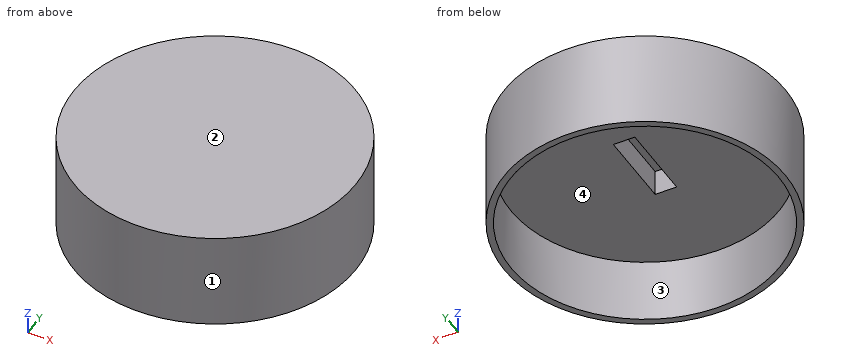
Autodesk Inventor part; units mm, degrees
ref_plane "YZ Plane" through (0, 0, 0) normal (1, 0, 0) x (0, 1, 0)
ref_plane "XZ Plane" through (0, 0, 0) normal (0, 1, 0) x (-1, 0, 0)
ref_plane "XY Plane" through (0, 0, 0) normal (0, 0, 1) x (1, 0, 0)
sketch "Esquisse1" plane through (0, 0, 0) normal (0, 0, 1) x (1, 0, 0)
  circle A0 centre (0, 0) radius 20.5
  circle A1 centre (0, 0) radius 21.5
  line L0 (0.7498, -6.187) -> (-0.7498, -6.187)
  line L1 (-0.7498, -6.187) -> (-0.7498, 6.187)
  line L2 (-0.7498, 6.187) -> (0.7498, 6.187)
  line L3 (0.7498, 6.187) -> (0.7498, -6.187)
  line L4 (0.7498, -6.187) -> (-0.7498, 6.187) construction
  line L5 (-0.7498, -6.187) -> (0.7498, 6.187) construction
  point P0 (20.5, 0)
  point P1 (21.5, 0)
  dimension "d0" = 41
  dimension "d1" = 43
  dimension "d16" = 1
extrude "Extrusion1" add sketch "Esquisse1" along normal blind 15 contours A1
sketch "Esquisse2" plane through (0, 0, 15) normal (0, 0, 1) x (1, 0, 0)
  circle A0 centre (0, 0) radius 20.5
extrude "Extrusion2" add sketch "Esquisse2" against normal blind 5
sketch "Esquisse3" plane through (0, 0, 10) normal (0, 0, -1) x (-1, 0, 0)
  line L0 (1.65, 6) -> (-1.65, 6)
  line L1 (-1.65, 6) -> (-1.65, -6)
  line L2 (-1.65, -6) -> (1.65, -6)
  line L3 (1.65, -6) -> (1.65, 6)
  line L4 (1.65, 6) -> (-1.65, -6) construction
  line L5 (-1.65, 6) -> (1.65, -6) construction
  point P0 (0, 0)
  dimension "d8" = 12
  dimension "d9" = 3.3
extrude "Extrusion3" cut sketch "Esquisse3" against normal blind 4
properties part number "Support pasApas"
Geometry check sheet. Reference: the model listing, model coordinates, mm. Face numbers are marked on the shaded views. Give positions to 0.01 mm unless a question says otherwise; leave off trailing zeros. Order: outer loops, then holes, each group sorted by start corner. A loop starts at its lowest first (then second) coordinate and runs counter-clockwise, first axis right, second up. Notation, with made-up numbers: (21, 12) - (42, 12) arc R14 cw to (42, 24) - close; hole circle Ø4 at (-33, 28). An arc over 180 degrees is marked (long way). Use one line per item in the form item = value.
1) Material ranges on probe 1 along X at (y, z) = (0.5, 8.5); probe 2 along Y at (x, z) = (0, 6.25); probe 3 along Z at (x, y) = (4.5, 15.5), recorded low to high. Write a range as from..to.
Working result:
probe_1 = -21.49..-20.49, 20.49..21.49
probe_2 = -21.5..-20.5, 20.5..21.5
probe_3 = 10..15
2) Sectioned sample at C-C (x = 0). Record the boundary of the cut face in (y, z), and give its area (3 significant figures).
Working result:
outline = (-21.5, 0) - (-20.5, 0) - (-20.5, 10) - (-6, 10) - (-6, 14) - (6, 14) - (6, 10) - (20.5, 10) - (20.5, 0) - (21.5, 0) - (21.5, 15) - (-21.5, 15) - close
area = 187 mm^2
3) Draft check along Y on the marked faces 1, 2, 3 and 4. Enter one of: released by +Y, released by -Y, zero draft, split by the parting line, or undercut.
Working result:
face_1 = split by the parting line
face_2 = zero draft
face_3 = undercut
face_4 = undercut
4) Sectioned sample at B-B (y = 0). Record the boundary of the cut face in (x, z), and give its area (3 significant figures).
Working result:
outline = (-21.5, 0) - (-20.5, 0) - (-20.5, 10) - (-1.65, 10) - (-1.65, 14) - (1.65, 14) - (1.65, 10) - (20.5, 10) - (20.5, 0) - (21.5, 0) - (21.5, 15) - (-21.5, 15) - close
area = 222 mm^2
5) Sectioned sample at A-A (z = 11.75). Record the boundary of the cut face in (x, y).
Working result:
outline = circle Ø43 at (0, 0); hole (-1.65, -6) - (1.65, -6) - (1.65, 6) - (-1.65, 6) - close
6) Depth check by flat-ended pin: pin 1 Ø3 at (y, z) = (-2.5, 12) entering from +X; pin 2 Ø8 at (y, z) = (15.5, 4) entering from -X; pin 3 Ø3.5 at (x, y) = (-0.5, 1.5) entering from -Z. Enter the tip coordinate at first touch or a pass-through.
Working result:
pin_1 = 21.48
pin_2 = -18.17
pin_3 = 10
7) Sectioned sample at D-D (z = 7.5). Record the boundary of the cut face in (x, y), and give its area (3 significant figures).
Working result:
outline = circle Ø43 at (0, 0); hole circle Ø41 at (0, 0)
area = 132 mm^2
